Geometry: final body of the model. Coordinates: model frame, mm. Face numbers are marked on the shaded views. A direction names the side the tool comes from. Round coordinates to 2 decimals unless told otherwise and drop trailing zeros. Order: outer loops, then holes, each group sorted by start corner. A loop starts at its lowest first (then second) coordinate and runs counter-clockwise, first axis right, second up. Notation, with made-up numbers: (-4.5, 89) - (15.5, 89) arc R22 cw to (15.5, 105) - close; hole circle Ø9 at (83.5, 37.5). An arc over 180 degrees is marked (long way). Put each result on its own line as item: value. Start each with the question number.
(1) Section B-B (x = 38.5). Output: boundary loops of the cut face in (y, z), and give its area (3 significant figures).
(2) Section A-A (y = 1.35). Output: boundary loops of the cut face in (x, z).
(3) Access query for the marked faces 1 and 2. Directions: +Z, -Z, +X, -X, +Y, -Y. A direction counts if a zero-diameter tool reaches every point of the face in a straight line with its end or side. Return the directions, or none.
(4) Material intervals for L1, parallel to Y at x = 30, z = -1; L2, parallel to Z at x = -8, y = -0.25; L3, parallel to X at y = 0.75, z = 23, sorted ascending. Write a range as [from, to].
(5) Pin query (flat end, axial travel): P1, Ø1.5, axis at x = -32.5, y = 0.5, coming from the -Z side; P2, Ø1.6, axis at x = -6.5, y = -1, coming from the +Z side; P3, Ø1, axis at y = -1, z = 3, coming from the -X side; P4, Ø1, axis at x = 19, z = -8.5, coming from the +Y side. Return the tip coordinate at first contact, or that it passes through.
(6) Section C-C (z = -4.5). Output: boundary loops of the cut face in (x, y).
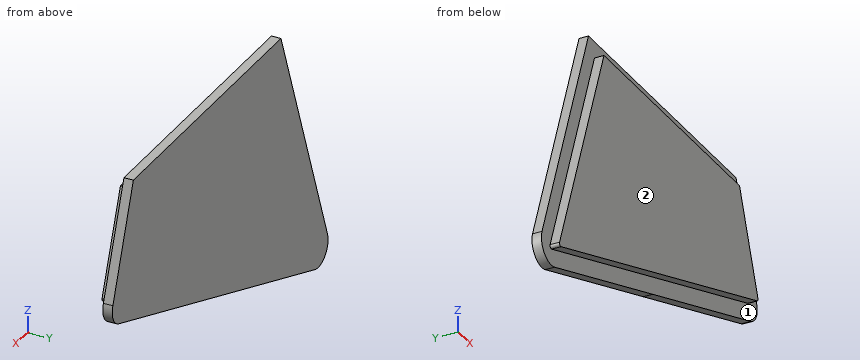
from build123d import *

# Parameters (mm, degrees)
BOSS_EXTRUDE1_DEPTH = 2
BOSS_EXTRUDE2_DEPTH = 2


with BuildPart() as part:
    # Sketch1 → Boss-Extrude1 (new body)
    with BuildSketch(Plane(origin=(0, 0, 0), x_dir=(1, 0, 0), z_dir=(0, 1, 0))):
        with BuildLine():
            Line((-24.718969723, -28.65368563), (35.281030277, -28.65368563))
            Line((35.281030277, -28.65368563), (43.623325522, -5.733417816))
            ThreePointArc((43.623325522, -5.733417816), (43.489786187, -2.674864196), (41.232635612, -0.60656676))
            Line((41.232635612, -0.60656676), (1.368080573, 13.902944676))
            Line((1.368080573, 13.902944676), (-38.496474466, 28.412456113))
            ThreePointArc((-38.496474466, 28.412456113), (-42.692982164, 27.482112755), (-43.623325522, 23.285605056))
            Line((-43.623325522, 23.285605056), (-24.718969723, -28.65368563))
        make_face()
    extrude(amount=BOSS_EXTRUDE1_DEPTH)

    # Sketch3 → Boss-Extrude2 (add)
    with BuildSketch(Plane.XZ):
        with BuildLine():
            Line((-22.26824334, 25.15368563), (-40.334401349, -24.482675558))
            ThreePointArc((-40.334401349, -24.482675558), (-40.21810843, -25.00723902), (-39.693544967, -25.12353194))
            Line((-39.693544967, -25.12353194), (40.035565111, 3.895490933))
            ThreePointArc((40.035565111, 3.895490933), (40.317708932, 4.154028112), (40.334401349, 4.536347315))
            Line((40.334401349, 4.536347315), (32.830303893, 25.15368563))
            Line((32.830303893, 25.15368563), (-22.26824334, 25.15368563))
        make_face()
    extrude(amount=BOSS_EXTRUDE2_DEPTH)


solid = part.part
Checks:
1. outline: (-2, 3.34) - (0, 3.34) - (0, -0.39) - (2, -0.39) - (2, 19.81) - (0, 19.81) - (0, 9.58) - (-2, 9.58) - close
1. area: 52.9 mm²
2. outline: (-43.62, -23.29) arc R4 ccw to (-38.5, -28.41) - (41.23, 0.61) arc R4 ccw to (43.62, 5.73) - (35.28, 28.65) - (-24.72, 28.65) - close
3. face 1: -Y
3. face 2: +Z, -Z, +X, -X, -Y
4. L1: y = [0, 2]
4. L2: z = [-13.59, 25.15]
4. L3: x = [-26.78, 37.34]
5. P1: stops at z = -26.5
5. P2: stops at z = 25.15
5. P3: stops at x = -30.51
5. P4: passes through
6. outline: (-36.79, 0) - (-33.06, 0) - (-33.06, -2) - (16.97, -2) - (16.97, 0) - (27.2, 0) - (27.2, 2) - (-36.79, 2) - close
